CAD build for the part. Positions are in the model's coordinates, mm. Face numbers are marked on the shaded views. A direction names the side the tool comes from. Give positions to 0.01 mm unless a question says otherwise; leave off trailing zeros. Loops run counter-clockwise (first coordinate to the right, second up) from the corner with the lowest first, then second, coordinate; pieces in that order, holes last. Notation, with made-up numbers: (31.25, 69.25) - (46.25, 69.25) arc R20 cw to (46.25, 91.25) - close; hole circle Ø3 at (53.5, 60). An arc over 180 degrees is marked (long way). Return JSON: item names as keys, results as strings.
from build123d import *

# Parameters (mm, degrees)
SKETCH1_W           = 25
SKETCH1_H           = 15
BOSS_EXTRUDE2_DEPTH = 22.5
CUT_EXTRUDE2_DEPTH  = 12.5


with BuildPart() as part:
    # Sketch1 → Boss-Extrude2 (new, symmetric)
    with BuildSketch(Plane(origin=(0, 0, 0), x_dir=(1, 0, 0), z_dir=(0, 1, 0))):
        Rectangle(SKETCH1_W, SKETCH1_H)
    extrude(amount=BOSS_EXTRUDE2_DEPTH, both=True)

    # Sketch5 → Cut-Extrude2 (cut)
    with BuildSketch(Plane.XY.offset(7.5)):
        Polygon((-8.5, 10.190598923), (-2.973720558, 7), (-5.598720558, 2.45336663), (-1.701606241, 0.20336663), (-2.951606241, -1.961696879), (-6.848720558, 0.288303121), (-12.5, -9.5), (-12.5, 24.790598923), (-8.5, 24.790598923), align=None)
    extrude(amount=-CUT_EXTRUDE2_DEPTH, mode=Mode.SUBTRACT)


solid = part.part
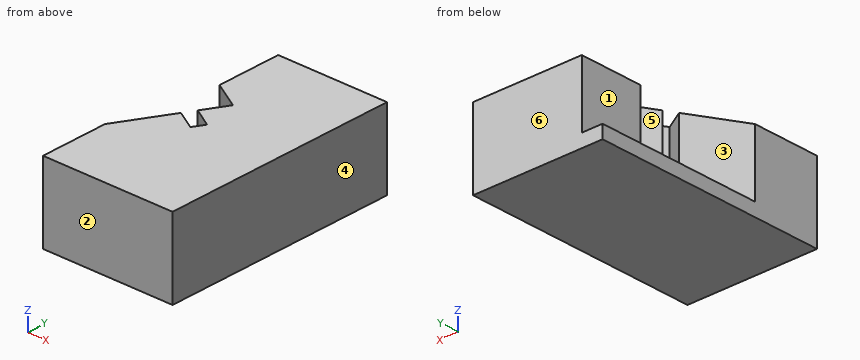
1. Cut at A-A, the plane z = 5. Write the cut outline in (x, y).
Values follow:
{"outline": "(-12.5, -22.5) - (12.5, -22.5) - (12.5, 22.5) - (-8.5, 22.5) - (-8.5, 10.19) - (-2.97, 7) - (-5.6, 2.45) - (-1.7, 0.2) - (-2.95, -1.96) - (-6.85, 0.29) - (-12.5, -9.5) - close"}
2. Drop a flat-ended pin along its axis: P1, Ø6, axis at y = 13.5, z = 1.5, coming from the -X side. Give the stop position or say it passes through.
Values follow:
{"P1": "stops at x = -8.5"}
3. Drill centre lines: probe 1 along Y at (x, z) = (-3.25, 3); probe 2 along Y at (x, z) = (-7.25, -3); probe 3 along X at (y, z) = (-0.5, 5). Where is each one in solid material? Low to high.
Values follow:
{"probe 1": "y = -22.5 to -1.79, 1.1 to 6.52, 7.16 to 22.5", "probe 2": "y = -22.5 to -0.41, 9.47 to 22.5", "probe 3": "x = -7.3 to -5.48, -2.11 to 12.5"}
4. Which spindle directions (+Z, -Z, +X, -X, +Y, -Y) get a long thin tool onto all of the face, cutting with end or side? Do the marked faces 1 and 2. Say none if no direction does.
Values follow:
{"face 1": "+Z, -X, +Y", "face 2": "+Z, -Z, +X, -X, -Y"}
5. Cut at B-B, the plane y = 11. Write the cut outline in (x, z), plus the area to 3 significant figures.
Values follow:
{"outline": "(-12.5, -7.5) - (12.5, -7.5) - (12.5, 7.5) - (-8.5, 7.5) - (-8.5, -5) - (-12.5, -5) - close", "area": "325 mm²"}
6. Cut at C-C, the plane x = -9.5. Write the cut outline in (y, z), plus the area to 3 significant figures.
Values follow:
{"outline": "(-22.5, -7.5) - (22.5, -7.5) - (22.5, -5) - (-4.3, -5) - (-4.3, 7.5) - (-22.5, 7.5) - close", "area": "340 mm²"}
7. Pull direction Y, two halves, no side cores. Call the marked faces 3, 4, 5 and 6: +Y half, -Y half, draft (parallel to the pull), parting line (faces both ways), or undercut.
Values follow:
{"face 3": "undercut", "face 4": "draft", "face 5": "undercut", "face 6": "+Y half"}
8. Cut at D-D, the plane x = -4.5. Write the cut outline in (y, z).
Values follow:
{"outline": "(-22.5, -7.5) - (22.5, -7.5) - (22.5, 7.5) - (7.88, 7.5) - (7.88, -5) - (4.36, -5) - (4.36, 7.5) - (1.82, 7.5) - (1.82, -5) - (-1.07, -5) - (-1.07, 7.5) - (-22.5, 7.5) - close"}
